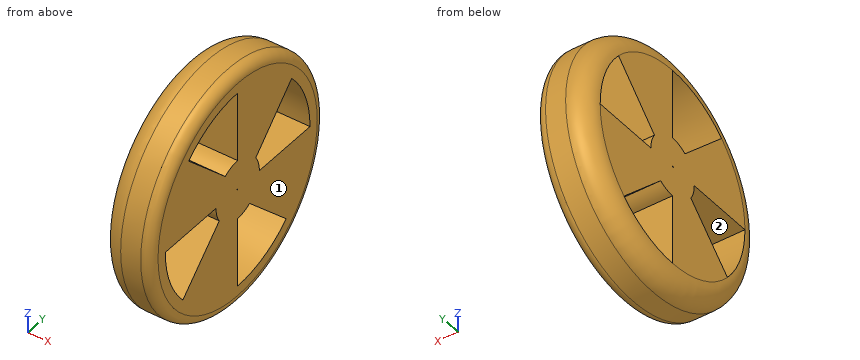
```python
from build123d import *

# Parameters (mm, degrees)
F0_R     = 60
F0_R_2   = 55
F1_DEPTH = 25
F2_R     = 5
F3_R     = 10
F4_DEPTH = 25
F5_DEPTH = 25


with BuildPart() as f1:
    # F0 (on Right) → F1 (new body)
    with BuildSketch(Plane.YZ):
        Circle(F0_R)
        Circle(F0_R_2, mode=Mode.SUBTRACT)
        Circle(F0_R_2)
        with BuildLine():
            ThreePointArc((37.3300225605, 33.2636350333), (46.7252668694, 17.7974558852), (50, 0))
            ThreePointArc((50, 0), (46.3547535543, -18.7413132657), (35.9505270831, -34.7499583085))
            ThreePointArc((35.9505270831, -34.7499583085), (34.7719029265, -35.9293023432), (33.5546123129, -37.0686928894))
            ThreePointArc((33.5546123129, -37.0686928894), (17.9800633415, -46.6553032595), (0, -50))
            ThreePointArc((0, -50), (-19.2409733878, -46.1495930978), (-35.5185237062, -35.1913977235))
            ThreePointArc((-35.5185237062, -35.1913977235), (-36.7306636988, -33.9243031505), (-37.8976277369, -32.6154842355))
            ThreePointArc((-37.8976277369, -32.6154842355), (-46.8768673593, -17.3942319916), (-50, 0))
            ThreePointArc((-50, 0), (-46.3446390349, 18.7663111114), (-35.9130226909, 34.7887165789))
            ThreePointArc((-35.9130226909, 34.7887165789), (-34.8991240146, 35.8057417605), (-33.8564359237, 36.7932296292))
            ThreePointArc((-33.8564359237, 36.7932296292), (-18.1705602354, 46.5814420207), (0, 50))
            ThreePointArc((0, 50), (1.5278005192, 49.9766528048), (3.054174244, 49.9066330229))
            ThreePointArc((3.054174244, 49.9066330229), (20.2598113498, 45.7114870035), (34.923788683, 35.7816850362))
            ThreePointArc((34.923788683, 35.7816850362), (36.148837516, 34.5436180248), (37.3300225605, 33.2636350333))
        make_face(mode=Mode.SUBTRACT)
        with BuildLine():
            ThreePointArc((-35.5185237062, -35.1913977235), (-19.2409733878, -46.1495930978), (0, -50))
            Line((0, -50), (0, -15))
            ThreePointArc((0, -15), (-5.9073859905, -13.7877768607), (-10.8599626488, -10.347038768))
            Line((-10.8599626488, -10.347038768), (-35.5185237062, -35.1913977235))
        make_face()
        with BuildLine():
            Line((-10.7607644181, 10.4501650292), (-35.9130226909, 34.7887165789))
            ThreePointArc((-35.9130226909, 34.7887165789), (-46.3446390349, 18.7663111114), (-50, 0))
            Line((-50, 0), (-15, 0))
            ThreePointArc((-15, 0), (-13.8998465148, 5.6386405156), (-10.7607644181, 10.4501650292))
        make_face()
        with BuildLine():
            ThreePointArc((35.9505270831, -34.7499583085), (46.3547535543, -18.7413132657), (50, 0))
            Line((50, 0), (15, 0))
            ThreePointArc((15, 0), (13.909961038, -5.6136426607), (10.7982688104, -10.4114067589))
            Line((10.7982688104, -10.4114067589), (35.9505270831, -34.7499583085))
        make_face()
        with BuildLine():
            Line((0, 15), (0, 50))
            ThreePointArc((0, 50), (-18.1705602354, 46.5814420207), (-33.8564359237, 36.7932296292))
            Line((-33.8564359237, 36.7932296292), (-8.5615410762, 12.3166559748))
            ThreePointArc((-8.5615410762, 12.3166559748), (-4.4860985488, 14.3134524071), (0, 15))
        make_face()
        with BuildLine():
            ThreePointArc((0, -50), (17.9800633415, -46.6553032595), (33.5546123129, -37.0686928894))
            Line((33.5546123129, -37.0686928894), (8.2159867451, -12.5498032576))
            ThreePointArc((8.2159867451, -12.5498032576), (4.2867791601, -14.3744051853), (0, -15))
            Line((0, -15), (0, -50))
        make_face()
        with BuildLine():
            Line((15, 0), (50, 0))
            ThreePointArc((50, 0), (46.7252668694, 17.7974558852), (37.3300225605, 33.2636350333))
            Line((37.3300225605, 33.2636350333), (12.5178824574, 8.264539841))
            ThreePointArc((12.5178824574, 8.264539841), (14.3660752619, 4.3146125631), (15, 0))
        make_face()
        with BuildLine():
            ThreePointArc((-50, 0), (-46.8768673593, -17.3942319916), (-37.8976277369, -32.6154842355))
            Line((-37.8976277369, -32.6154842355), (-12.6869769146, -8.0025381453))
            ThreePointArc((-12.6869769146, -8.0025381453), (-14.4101466634, -4.165053798), (-15, 0))
            Line((-15, 0), (-50, 0))
        make_face()
        with BuildLine():
            Line((10.2652276257, 10.9373260806), (34.923788683, 35.7816850362))
            ThreePointArc((34.923788683, 35.7816850362), (20.2598113498, 45.7114870035), (3.054174244, 49.9066330229))
            Line((3.054174244, 49.9066330229), (3.054174244, 14.6857761009))
            ThreePointArc((3.054174244, 14.6857761009), (6.9184055916, 13.309232287), (10.2652276257, 10.9373260806))
        make_face()
        with BuildLine():
            Line((12.5178824574, 8.264539841), (37.3300225605, 33.2636350333))
            ThreePointArc((37.3300225605, 33.2636350333), (36.148837516, 34.5436180248), (34.923788683, 35.7816850362))
            Line((34.923788683, 35.7816850362), (10.2652276257, 10.9373260806))
            ThreePointArc((10.2652276257, 10.9373260806), (11.4696762306, 9.666774393), (12.5178824574, 8.264539841))
        make_face()
        with BuildLine():
            ThreePointArc((33.5546123129, -37.0686928894), (34.7719029265, -35.9293023432), (35.9505270831, -34.7499583085))
            Line((35.9505270831, -34.7499583085), (10.7982688104, -10.4114067589))
            ThreePointArc((10.7982688104, -10.4114067589), (9.5670613815, -11.5529795517), (8.2159867451, -12.5498032576))
            Line((8.2159867451, -12.5498032576), (33.5546123129, -37.0686928894))
        make_face()
        with BuildLine():
            ThreePointArc((-37.8976277369, -32.6154842355), (-36.7306636988, -33.9243031505), (-35.5185237062, -35.1913977235))
            Line((-35.5185237062, -35.1913977235), (-10.8599626488, -10.347038768))
            ThreePointArc((-10.8599626488, -10.347038768), (-11.8316846431, -9.2201539307), (-12.6869769146, -8.0025381453))
            Line((-12.6869769146, -8.0025381453), (-37.8976277369, -32.6154842355))
        make_face()
        with BuildLine():
            Line((3.054174244, 14.6857761009), (3.054174244, 49.9066330229))
            ThreePointArc((3.054174244, 49.9066330229), (1.5278005192, 49.9766528048), (0, 50))
            Line((0, 50), (0, 15))
            ThreePointArc((0, 15), (1.5351479547, 14.9212372395), (3.054174244, 14.6857761009))
        make_face()
        with BuildLine():
            Line((-8.5615410762, 12.3166559748), (-33.8564359237, 36.7932296292))
            ThreePointArc((-33.8564359237, 36.7932296292), (-34.8991240146, 35.8057417605), (-35.9130226909, 34.7887165789))
            Line((-35.9130226909, 34.7887165789), (-10.7607644181, 10.4501650292))
            ThreePointArc((-10.7607644181, 10.4501650292), (-9.7061227849, 11.4363971811), (-8.5615410762, 12.3166559748))
        make_face()
    extrude(amount=F1_DEPTH)

    # F2
    f2_edges = [f1.edges().sort_by_distance(p)[0] for p in [
        (25, -60, 0),
    ]]
    fillet(f2_edges, radius=F2_R)

    # F3
    f3_edges = [f1.edges().sort_by_distance(p)[0] for p in [
        (0, -60, 0),
    ]]
    fillet(f3_edges, radius=F3_R)

    # F0 (on Right) → F4 (cut, through all)
    with BuildSketch(Plane.YZ):
        with BuildLine():
            Line((0, 15), (0, 50))
            ThreePointArc((0, 50), (-18.1705602354, 46.5814420207), (-33.8564359237, 36.7932296292))
            Line((-33.8564359237, 36.7932296292), (-8.5615410762, 12.3166559748))
            ThreePointArc((-8.5615410762, 12.3166559748), (-4.4860985488, 14.3134524071), (0, 15))
        make_face()
        with BuildLine():
            ThreePointArc((-50, 0), (-46.8768673593, -17.3942319916), (-37.8976277369, -32.6154842355))
            Line((-37.8976277369, -32.6154842355), (-12.6869769146, -8.0025381453))
            ThreePointArc((-12.6869769146, -8.0025381453), (-14.4101466634, -4.165053798), (-15, 0))
            Line((-15, 0), (-50, 0))
        make_face()
        with BuildLine():
            ThreePointArc((0, -50), (17.9800633415, -46.6553032595), (33.5546123129, -37.0686928894))
            Line((33.5546123129, -37.0686928894), (8.2159867451, -12.5498032576))
            ThreePointArc((8.2159867451, -12.5498032576), (4.2867791601, -14.3744051853), (0, -15))
            Line((0, -15), (0, -50))
        make_face()
        with BuildLine():
            Line((15, 0), (50, 0))
            ThreePointArc((50, 0), (46.7252668694, 17.7974558852), (37.3300225605, 33.2636350333))
            Line((37.3300225605, 33.2636350333), (12.5178824574, 8.264539841))
            ThreePointArc((12.5178824574, 8.264539841), (14.3660752619, 4.3146125631), (15, 0))
        make_face()
    extrude(amount=F4_DEPTH, mode=Mode.SUBTRACT)

    # F0 (on Right) → F5 (join)
    with BuildSketch(Plane.YZ):
        with BuildLine():
            ThreePointArc((10.7982688104, -10.4114067589), (13.909961038, -5.6136426607), (15, 0))
            ThreePointArc((15, 0), (14.3660752619, 4.3146125631), (12.5178824574, 8.264539841))
            ThreePointArc((12.5178824574, 8.264539841), (11.4696762306, 9.666774393), (10.2652276257, 10.9373260806))
            ThreePointArc((10.2652276257, 10.9373260806), (6.9184055916, 13.309232287), (3.054174244, 14.6857761009))
            ThreePointArc((3.054174244, 14.6857761009), (1.5351479547, 14.9212372395), (0, 15))
            ThreePointArc((0, 15), (-4.4860985488, 14.3134524071), (-8.5615410762, 12.3166559748))
            ThreePointArc((-8.5615410762, 12.3166559748), (-9.7061227849, 11.4363971811), (-10.7607644181, 10.4501650292))
            ThreePointArc((-10.7607644181, 10.4501650292), (-13.8998465148, 5.6386405156), (-15, 0))
            ThreePointArc((-15, 0), (-14.4101466634, -4.165053798), (-12.6869769146, -8.0025381453))
            ThreePointArc((-12.6869769146, -8.0025381453), (-11.8316846431, -9.2201539307), (-10.8599626488, -10.347038768))
            ThreePointArc((-10.8599626488, -10.347038768), (-5.9073859905, -13.7877768607), (0, -15))
            ThreePointArc((0, -15), (4.2867791601, -14.3744051853), (8.2159867451, -12.5498032576))
            ThreePointArc((8.2159867451, -12.5498032576), (9.5670613815, -11.5529795517), (10.7982688104, -10.4114067589))
        make_face()
        Polygon((-0.2821140827, 0.3105120171), (0, 0.5947517795), (0, 0.0375246745), (0.0387792307, 0), (0, 0), (-0.5903039437, 0), align=None, mode=Mode.SUBTRACT)
    extrude(amount=F5_DEPTH)


solid = f1.part
```
Geometry check sheet. Reference: the model listing, model coordinates, mm. Face numbers are marked on the shaded views. A direction names the side the tool comes from. Coordinates: 2 decimals unless noted, no trailing zeros. Order: outer loops, then holes, each group sorted by start corner. A loop starts at its lowest first (then second) coordinate and runs counter-clockwise, first axis right, second up.
Item 1: Tool access check on the marked faces 1 and 2. Record the directions out of +Z, -Z, +X, -X, +Y, -Y that give a thin tool (end or side, any length) a straight path to the whole face; none if there is none.
Item 2: Section check B-B (z = -20). Count the separate pieces of the cut face and the enclosed holes in it, plus the area to 3 significant figures.
Item 3: Scan lines: line 1 along Z through (x, y) = (21.25, -22); line 2 along Z through (x, y) = (22.75, -27.5); line 3 along Y through (x, z) = (22.75, -15.5). Record each from-to range of solid material in increasing order.
Item 4: Section check A-A (x = 5.5). Enter the section's corners in (y, z).
Item 5: Depth check by flat-ended pin: pin 1 (6 mm diameter, centred on x = 7.5, y = 26.5, fed in from -Z); pin 2 (1.5 mm diameter, centred on x = 6.5, z = 21, fed in from -Y); pin 3 (3 mm diameter, centred on y = -25.5, z = 46.5, fed in from -X). Enter the tip coordinate at first touch or a pass-through.
Check sheet entries:
1. face 1: +Z, -Z, +X, +Y, -Y
1. face 2: +X, -X
2. separate pieces: 3
2. enclosed holes: 0
2. area: 1,850 mm2
3. line 1: z = -55.65 to -17.09, 0 to 25.32, 44.9 to 55.65
3. line 2: z = -52.4 to -22.46, 0 to 30.64, 41.76 to 52.4
3. line 3: y = -57.11 to -47.54, -20.37 to 0, 11.26 to 57.11
4. outline: circle Ø117.86 at (0, 0); hole (-50, 0) arc R50 ccw to (-37.9, -32.62) - (-12.69, -8) arc R15 cw to (-15, 0) - close; hole (-33.86, 36.79) - (-8.56, 12.32) arc R15 cw to (0, 15) - (0, 50) arc R50 ccw to start; hole (-0.59, 0) - (0.04, 0) - (0, 0.04) - (0, 0.59) - close; hole (0, -50) arc R50 ccw to (33.55, -37.07) - (8.22, -12.55) arc R15 cw to (0, -15) - close; hole (12.52, 8.26) arc R15 cw to (15, 0) - (50, 0) arc R50 ccw to (37.33, 33.26) - close
5. pin 1: stops at z = -55.01
5. pin 2: stops at y = -55.92
5. pin 3: stops at x = 0.12
